Job drawing, mm, ordinate dimensions from the low corner. One solid piece. A direction names the side the tool comes from. Round coordinates to 2 decimals unless told otherwise and drop trailing zeros. Order: outer loops, then holes, each group sorted by start corner. A loop starts at its lowest first (then second) coordinate and runs counter-clockwise, first axis right, second up. Notation, with made-up numbers: (48, 70) -> (52, 70) arc R13 ccw to (52, 78) -> close; hole circle Ø9 at (64.5, 55.5). An arc over 180 degrees is marked (long way). Write item = value, one per line.
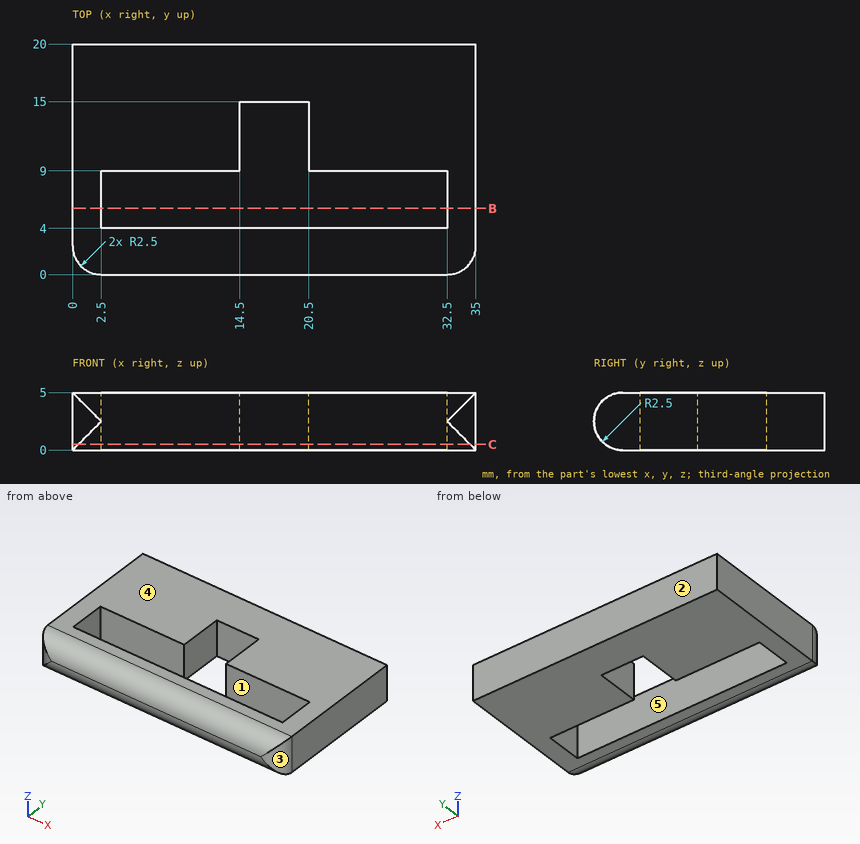
Q1. Mould opens along Y. For the marked faces 1, 2 and 3 say: released by +Y, released by -Y, zero draft, split by the parting line, or undercut.
Check values:
face_1 = undercut
face_2 = released by +Y
face_3 = released by -Y
Q2. Probe probe 1 along X at (y, z) = (8, 0.7); probe 2 along X at (y, z) = (10.75, 1.1); probe 3 along Y at (x, z) = (3, 2.45). List the from-to ranges inside material, lowest first.
Check values:
probe_1 = 0 to 2.5, 32.5 to 35
probe_2 = 0 to 14.5, 20.5 to 35
probe_3 = 0 to 4, 9 to 20
Q3. Cut at C-C, the plane z = 0.5. List the corners of the cut face in (x, y), and give its area (3 significant figures).
Check values:
outline = (0, 2.5) arc R2.5 ccw to (0.5, 1) -> (34.5, 1) arc R2.5 ccw to (35, 2.5) -> (35, 20) -> (0, 20) -> close; hole (2.5, 4) -> (32.5, 4) -> (32.5, 9) -> (20.5, 9) -> (20.5, 15) -> (14.5, 15) -> (14.5, 9) -> (2.5, 9) -> close
area = 479 mm²
Q4. Cut at B-B, the plane y = 5.75. List the corners of the cut face in (x, z).
Check values:
outline = (0, 0) -> (2.5, 0) -> (2.5, 5) -> (0, 5) -> close; (32.5, 0) -> (35, 0) -> (35, 5) -> (32.5, 5) -> close
Q5. Which spindle directions (+Z, -Z, +X, -X, +Y, -Y) get a long thin tool onto all of the face, cutting with end or side? Do the marked faces 4 and 5. Say none if no direction does.
Check values:
face_4 = +Z, +X, -X, +Y, -Y
face_5 = +Z, -Z
